Can you work these out from the model? Positions are in its coordinate system, mm. Face numbers are marked on the shaded views. Round coordinates to 2 decimals unless told otherwise and drop trailing zeros. Write each loop counter-clockwise with the first axis right and the second up, starting at its lowest first coordinate (ties: lowest second). Pieces come first, ordered by that corner, then holes.
Q1. If we section it at D-D (z = 36): Please give me the cut outline in (x, y), plus the area to 3 significant figures.
Q2. Please list where these lines run through material, in increasing order: line 1 along X through (y, z) = (12.5, -6); line 2 along Y through (x, z) = (-22, -17); line 3 along Z through (x, y) = (2, 13).
Q3. If we section it at A-A (x = 0): Please give me the cut outline in (y, z) (1 decimal), plus the area to 3 significant figures.
Q4. If we section it at C-C (y = 1): Please give me the cut outline in (x, z) (3 decimals), plus the area to 3 significant figures.
Q5. We'd pull the mould along X, two halves only. Please class the marked faces 1, 2 and 3: +X half, -X half, draft (parallel to the pull), parting line (faces both ways), or undercut.
Q6. If we section it at B-B (z = 0): Please give me the cut outline in (x, y) (1 decimal), plus the area to 3 significant figures.
Q7. I'm going to push flat-ended pins straight in: pin 1 Ø8 at (y, z) = (5.5, 12.5) entering from +X; pin 2 Ø8.5 at (y, z) = (11, 0) entering from -X; pin 3 Ø5 at (x, y) = (31, 2.5) entering from -Z. Where does each tip first touch, or does it pass through?
from build123d import *

# Parameters (mm, degrees)
SKETCH1_R           = 41.275
BOSS_EXTRUDE1_DEPTH = 4.7625
SKETCH2_W           = 18
SKETCH2_H           = 18
BOSS_EXTRUDE2_DEPTH = 5.334
FILLET1_R           = 2.54
BOSS_EXTRUDE3_DEPTH = 5.08


with BuildPart() as part:
    # Sketch1 → Boss-Extrude1 (new body)
    with BuildSketch(Plane(origin=(0, 0, 0), x_dir=(1, 0, 0), z_dir=(0, 1, 0))):
        Circle(SKETCH1_R)
    extrude(amount=BOSS_EXTRUDE1_DEPTH)

    # Sketch2 → Boss-Extrude2 (add)
    with BuildSketch(Plane(origin=(0, 4.7625, 0), x_dir=(1, 0, 0), z_dir=(0, 1, 0))):
        Rectangle(SKETCH2_W, SKETCH2_H)
    extrude(amount=BOSS_EXTRUDE2_DEPTH)

    # Fillet1
    fillet1_edges = [part.edges().sort_by_distance(p)[0] for p in [
        (9, 4.7625, 0),
        (0, 4.7625, -9),
        (-9, 4.7625, 0),
        (0, 4.7625, 9),
    ]]
    fillet(fillet1_edges, radius=FILLET1_R)

    # Sketch3 → Boss-Extrude3 (add)
    with BuildSketch(Plane(origin=(0, 10.0965, 0), x_dir=(1, 0, 0), z_dir=(0, 1, 0))):
        Polygon((-9, -9), (9, -9), (9, 9), (6.5, 9), (6.5, -5.5), (-6.5, -5.5), (-6.5, 9), (-9, 9), align=None)
    extrude(amount=BOSS_EXTRUDE3_DEPTH)


solid = part.part
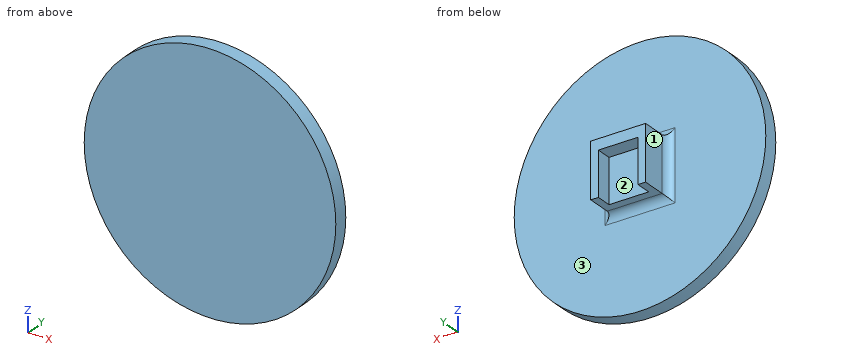
A:
1. outline: (-20.19, 0) - (20.19, 0) - (20.19, 4.76) - (-20.19, 4.76) - close
1. area: 192 mm2
2. line 1: x = -9 to -6.5, 6.5 to 9
2. line 2: y = 0 to 4.76
2. line 3: z = 5.5 to 9
3. outline: (0, -41.3) - (4.8, -41.3) - (4.8, -11.5) arc R2.5 cw to (7.3, -9) - (10.1, -9) - (10.1, 5.5) - (15.2, 5.5) - (15.2, 9) - (7.3, 9) arc R2.5 cw to (4.8, 11.5) - (4.8, 41.3) - (0, 41.3) - close
3. area: 510 mm2
4. outline: circle Ø82.55 at (0, 0)
4. area: 5,350 mm2
5. face 1: -X half
5. face 2: undercut
5. face 3: draft
6. outline: (-41.3, 0) - (41.3, 0) - (41.3, 4.8) - (11.5, 4.8) arc R2.5 cw to (9, 7.3) - (9, 15.2) - (6.5, 15.2) - (6.5, 10.1) - (-6.5, 10.1) - (-6.5, 15.2) - (-9, 15.2) - (-9, 7.3) arc R2.5 cw to (-11.5, 4.8) - (-41.3, 4.8) - close
6. area: 517 mm2
7. pin 1: stops at x = 40.38
7. pin 2: stops at x = -9.06
7. pin 3: stops at z = -29.86
